from build123d import *

# Parameters (mm, degrees)
CROQUIS1_R              = 10
CROQUIS1_R_2            = 4.05
SALIENTE_EXTRUIR1_DEPTH = 26.4
CROQUIS2_R              = 7.05
CROQUIS2_R_2            = 4.05
SALIENTE_EXTRUIR2_DEPTH = 1.75
CROQUIS3_R              = 7.05
CROQUIS3_R_2            = 4.05
SALIENTE_EXTRUIR3_DEPTH = 1.75


with BuildPart() as part:
    # Croquis1 → Saliente-Extruir1 (new body)
    with BuildSketch(Plane.XY):
        Circle(CROQUIS1_R)
        Circle(CROQUIS1_R_2, mode=Mode.SUBTRACT)
    extrude(amount=SALIENTE_EXTRUIR1_DEPTH)

    # Croquis2 → Saliente-Extruir2 (add)
    with BuildSketch(Plane.XY.offset(26.4)):
        Circle(CROQUIS2_R)
        Circle(CROQUIS2_R_2, mode=Mode.SUBTRACT)
    extrude(amount=SALIENTE_EXTRUIR2_DEPTH)

    # Croquis3 → Saliente-Extruir3 (add)
    with BuildSketch(Plane(origin=(0, 0, 0), x_dir=(-1, 0, 0), z_dir=(0, 0, -1))):
        Circle(CROQUIS3_R)
        Circle(CROQUIS3_R_2, mode=Mode.SUBTRACT)
    extrude(amount=SALIENTE_EXTRUIR3_DEPTH)


solid = part.part
Work out the finished part from the listing and answer in its coordinate system (mm). A direction names the side the tool comes from. Give positions to 0.01 mm unless a question says otherwise; leave off trailing zeros. Loops run counter-clockwise (first coordinate to the right, second up) from the corner with the lowest first, then second, coordinate; pieces in that order, holes last. Notation, with made-up numbers: (70.5, 89) -> (113.5, 89) arc R26 ccw to (113.5, 103) -> close; hole circle Ø9 at (51, 16). An arc over 180 degrees is marked (long way). Use a Markdown table: item, result. Add a question column.
1. Section C-C on z = 5.25 is taken. Determine the outline of the cut face in (x, y), and give its area (3 significant figures).
2. Section A-A on y = 0 is taken. Determine the outline of the cut face in (x, z).
3. Flat-ended cylindrical pins translate along their axes: pin 1 Ø12 at (x, z) = (-1, 16.5) entering from -Y; pin 2 Ø5 at (y, z) = (-7.5, 23.5) entering from -X; pin 3 Ø7.5 at (x, y) = (0, 0) entering from +Z; pin 4 Ø10 at (y, z) = (7.5, 25) entering from -X. Find the tip coordinate at first contact, or state that the pin passes through.
4. Find the intervals of material crossed by probe 1 along Y at (x, z) = (0, -0.7); probe 2 along Y at (x, z) = (0, 15.5); probe 3 along X at (y, z) = (0.25, 2), in increasing order.
5. Section D-D on y = -5.25 is taken. Determine the outline of the cut face in (x, z).
6. Determine the mould class of faces 1 (the cylindrical face through (-2.17, -9.76, 13.02)), 2 (the flat face through (-3, -3, -1.75)), 3 (the flat face through (3, -3, 28.15)) for opening direction Z: released by +Z, released by -Z, zero draft, split by the parting line, or undercut.
7. For faces 4 (the flat face through (-7, -2, 0)), 5 (the flat face through (-7, -2, 26.4)), determine the directions among +Z, -Z, +X, -X, +Y, -Y from which every point of the face is accessible in a straight line to the end or side of a thin tool.
Results below:
| question | item | result |
|---|---|---|
| 1 | outline | circle Ø20 at (0, 0); hole circle Ø8.1 at (0, 0) |
| 1 | area | 263 mm^2 |
| 2 | outline | (-10, 0) -> (-7.05, 0) -> (-7.05, -1.75) -> (-4.05, -1.75) -> (-4.05, 28.15) -> (-7.05, 28.15) -> (-7.05, 26.4) -> (-10, 26.4) -> close; (4.05, -1.75) -> (7.05, -1.75) -> (7.05, 0) -> (10, 0) -> (10, 26.4) -> (7.05, 26.4) -> (7.05, 28.15) -> (4.05, 28.15) -> close |
| 3 | pin 1 | stops at y = -10 |
| 3 | pin 2 | stops at x = -8.66 |
| 3 | pin 3 | passes through |
| 3 | pin 4 | stops at x = -9.68 |
| 4 | probe 1 | y = -7.05 to -4.05, 4.05 to 7.05 |
| 4 | probe 2 | y = -10 to -4.05, 4.05 to 10 |
| 4 | probe 3 | x = -10 to -4.04, 4.04 to 10 |
| 5 | outline | (-8.51, 0) -> (-4.71, 0) -> (-4.71, -1.75) -> (4.71, -1.75) -> (4.71, 0) -> (8.51, 0) -> (8.51, 26.4) -> (4.71, 26.4) -> (4.71, 28.15) -> (-4.71, 28.15) -> (-4.71, 26.4) -> (-8.51, 26.4) -> close |
| 6 | face 1 | zero draft |
| 6 | face 2 | released by -Z |
| 6 | face 3 | released by +Z |
| 7 | face 4 | -Z |
| 7 | face 5 | +Z |
